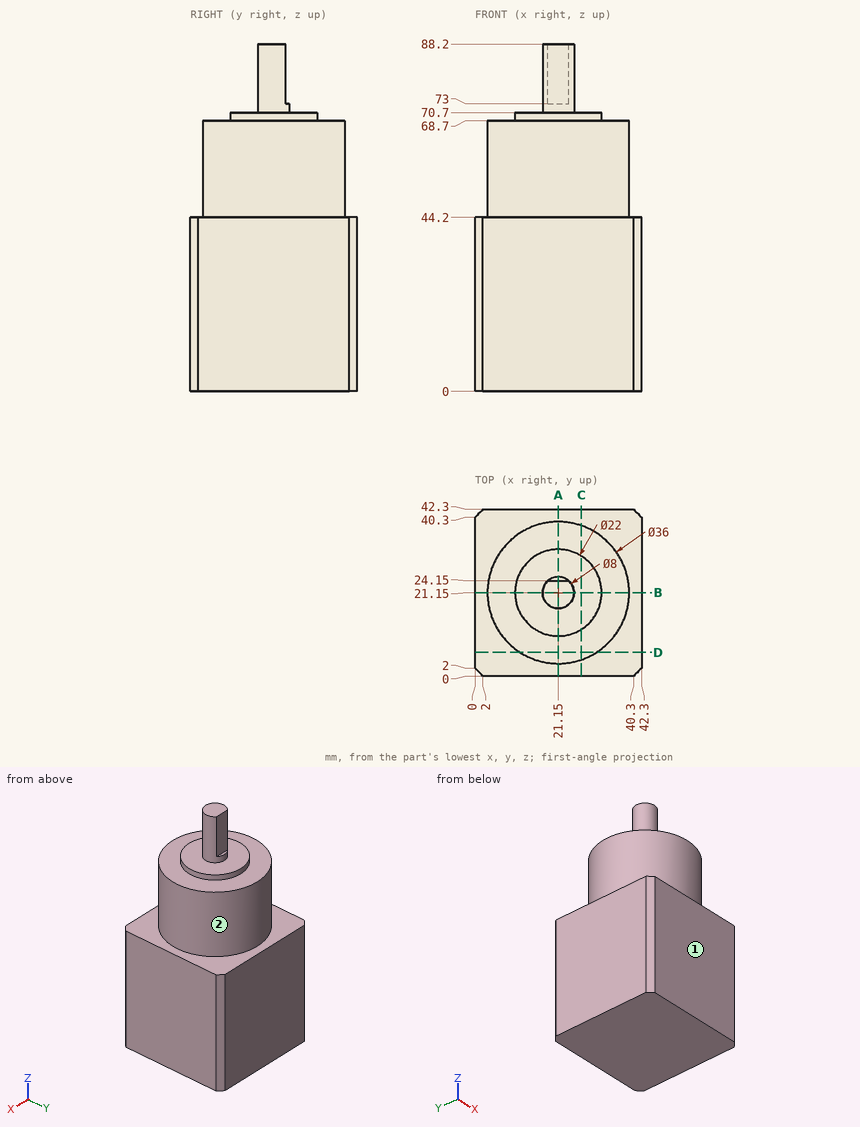
Job drawing, mm, ordinate dimensions from the low corner. One solid piece. A direction names the side the tool comes from. Give positions to 0.01 mm unless a question says otherwise; leave off trailing zeros. Loops run counter-clockwise (first coordinate to the right, second up) from the corner with the lowest first, then second, coordinate; pieces in that order, holes last. Notation, with made-up numbers: (41.25, 44) -> (100.25, 44) arc R32 cw to (100.25, 78) -> close; hole circle Ø10 at (12, -27). An arc over 180 degrees is marked (long way). Write each question's results on one line, items separated by ' | '.
(1) Flat gauge pins, fed straight in: pin 1 Ø1.6 at (x, z) = (22, 84) entering from +Y; pin 2 Ø3 at (x, y) = (28.5, 23) entering from +Z; pin 3 Ø1 at (x, z) = (28, 67.5) entering from -Y. Where does each tip first touch, or does it go through?
Geometry results:
pin 1: stops at y = 24.15 | pin 2: stops at z = 70.7 | pin 3: stops at y = 4.31
(2) Cut at C-C on x = 27. List the corners of the cut face in (y, z).
Geometry results:
outline: (0, 0) -> (42.3, 0) -> (42.3, 44.2) -> (38.17, 44.2) -> (38.17, 68.7) -> (30.47, 68.7) -> (30.47, 70.7) -> (11.83, 70.7) -> (11.83, 68.7) -> (4.13, 68.7) -> (4.13, 44.2) -> (0, 44.2) -> close
(3) Probe line 1 along Z through (x, y) = (4, 26); line 2 along Z through (x, y) = (17, 14.5); line 3 along Y through (x, z) = (34, 50.5). List the from-to ranges inside material, lowest first.
Geometry results:
line 1: z = 0 to 68.7 | line 2: z = 0 to 70.7 | line 3: y = 8.55 to 33.75
(4) Cut at B-B on y = 21.15. List the corners of the cut face in (x, z).
Geometry results:
outline: (0, 0) -> (42.3, 0) -> (42.3, 44.2) -> (39.15, 44.2) -> (39.15, 68.7) -> (32.15, 68.7) -> (32.15, 70.7) -> (25.15, 70.7) -> (25.15, 88.2) -> (17.15, 88.2) -> (17.15, 70.7) -> (10.15, 70.7) -> (10.15, 68.7) -> (3.15, 68.7) -> (3.15, 44.2) -> (0, 44.2) -> close
(5) Cut at D-D on y = 6. List the corners of the cut face in (x, z).
Geometry results:
outline: (0, 0) -> (42.3, 0) -> (42.3, 44.2) -> (30.87, 44.2) -> (30.87, 68.7) -> (11.43, 68.7) -> (11.43, 44.2) -> (0, 44.2) -> close
(6) Cut at A-A on x = 21.15. List the corners of the cut face in (y, z), and give its area (3 significant figures).
Geometry results:
outline: (0, 0) -> (42.3, 0) -> (42.3, 44.2) -> (39.15, 44.2) -> (39.15, 68.7) -> (32.15, 68.7) -> (32.15, 70.7) -> (25.15, 70.7) -> (25.15, 73) -> (24.15, 73) -> (24.15, 88.2) -> (17.15, 88.2) -> (17.15, 70.7) -> (10.15, 70.7) -> (10.15, 68.7) -> (3.15, 68.7) -> (3.15, 44.2) -> (0, 44.2) -> close | area: 2,920 mm²
(7) Tool access for the marked faces 1 and 2: list every direction of +Z, -Z, +X, -X, +Y, -Y with a clear straight run to the whole face (end or side of a thin tool).
Geometry results:
face 1: +Z, -Z, +X, -X, -Y | face 2: +Z
